Geometry: final body of the model. Coordinates: model frame, mm. A direction names the side the tool comes from. Coordinates: 2 decimals unless noted, no trailing zeros. Order: outer loops, then holes, each group sorted by start corner. A loop starts at its lowest first (then second) coordinate and runs counter-clockwise, first axis right, second up. Notation, with made-up numbers: M 65.5,-5.75 L 72.5,-5.75 A37 ccw 72.5,31.25 Z; hole C 53,60 d1. An arc over 180 degrees is marked long. One line per question, with ' | ' between items.
from build123d import *

# Parameters (mm, degrees)
SKETCH1_W   = 2
SKETCH1_H   = 44.5
ESQUISSE1_W = 0.574838605
ESQUISSE1_H = 0.64
ESQUISSE3_W = 1.093459546
ESQUISSE3_H = 0.64


with BuildPart() as part:
    # Sketch1 → Revolve1 (revolve)
    with BuildSketch(Plane.XY):
        with Locations((1, 22.25)):
            Rectangle(SKETCH1_W, SKETCH1_H)
    revolve(axis=Axis((0, 0, 0), (0, 1, 0)))

    # Esquisse1 → Enlèvement de matière-Révolution1 (revolve, cut)
    with BuildSketch(Plane.XY):
        with Locations((1.887419303, 43.18)):
            Rectangle(ESQUISSE1_W, ESQUISSE1_H)
    revolve(axis=Axis((0, 44.5, 0), (0, -1, 0)), mode=Mode.SUBTRACT)

    # Esquisse3 → Enlèvement de matière-Révolution3 (revolve, cut)
    with BuildSketch(Plane.XY):
        with Locations((2.146729773, 1.32)):
            Rectangle(ESQUISSE3_W, ESQUISSE3_H)
    revolve(axis=Axis((0, 44.5, 0), (0, -1, 0)), mode=Mode.SUBTRACT)


solid = part.part
1. Section B-B, the plane y = 6. Output: boundary loops of the cut face in (x, z).
Response values:
outline: C 0,0 d4
2. Section C-C, the plane z = -0.75. Output: boundary loops of the cut face in (x, y), and give its area (3 significant figures).
Response values:
outline: M -1.85,0 L 1.85,0 L 1.85,1 L 1.41,1 L 1.41,1.64 L 1.85,1.64 L 1.85,42.86 L 1.41,42.86 L 1.41,43.5 L 1.85,43.5 L 1.85,44.5 L -1.85,44.5 L -1.85,43.5 L -1.41,43.5 L -1.41,42.86 L -1.85,42.86 L -1.85,1.64 L -1.41,1.64 L -1.41,1 L -1.85,1 Z | area: 164 mm^2
3. Access query for faces 1 (the face through (-1.27, 1.32, -0.97)), 2 (the face through (0, 44, 2)). Directions: +Z, -Z, +X, -X, +Y, -Y. A direction counts if a zero-diameter tool reaches every point of the face in a straight line with its end or side. Return the directions, or none.
Response values:
face 1: none | face 2: +Y, -Y
4. Section A-A, the plane x = 0.95. Output: boundary loops of the cut face in (y, z).
Response values:
outline: M 0,-1.76 L 1,-1.76 L 1,-1.29 L 1.64,-1.29 L 1.64,-1.76 L 42.86,-1.76 L 42.86,-1.29 L 43.5,-1.29 L 43.5,-1.76 L 44.5,-1.76 L 44.5,1.76 L 43.5,1.76 L 43.5,1.29 L 42.86,1.29 L 42.86,1.76 L 1.64,1.76 L 1.64,1.29 L 1,1.29 L 1,1.76 L 0,1.76 Z
5. Material intervals for line 1 (Y direction, x = -1.25, z = -1.15); line 2 (X direction, y = 14, z = -0.75); line 3 (X direction, y = 11, z = 1), sorted ascending. Write a range as [from, to].
Response values:
line 1: y = [0, 1], [1.64, 42.86], [43.5, 44.5] | line 2: x = [-1.85, 1.85] | line 3: x = [-1.73, 1.73]
6. Pin query (flat end, axial travel): P1, Ø1, axis at x = -1, y = 29.5, coming from the +Z side. Return the tip coordinate at first contact, or that it passes through.
Response values:
P1: stops at z = 1.94
7. Draft query along Y for faces 3 (the face through (0, 44.5, 0)), 4 (the face through (0, 23, 2)), 5 (the face through (1.526, 43.184, 0.481)). Return one class per face: pulls with the +Y half, pulls with the -Y half, needs draft (parallel to the pull), parting line crosses it, or undercut.
Response values:
face 3: pulls with the +Y half | face 4: needs draft | face 5: undercut
